Build history of the part. All positions in model axes, mm. Face numbers are marked on the shaded views. A direction names the side the tool comes from. Round coordinates to 2 decimals unless told otherwise and drop trailing zeros. Loops run counter-clockwise (first coordinate to the right, second up) from the corner with the lowest first, then second, coordinate; pieces in that order, holes last. Notation, with made-up numbers: (75, -13) - (102, -13) arc R25 cw to (102, 25) - close; hole circle Ø10 at (-7.75, -20). An arc over 180 degrees is marked (long way). Use one line per item in the form item = value. Start each with the question number.
Q1. Drill centre lines: line 1 (Y direction, x = 9, z = -1); line 2 (Z direction, x = 18, y = 40); line 3 (Y direction, x = 23, z = 0). Where is each one in solid material? Low to high.
Q2. Mould opens along X. For the marked faces 3 and 4 say: released by +X, released by -X, zero draft, split by the parting line, or undercut.
Q3. Saw through at A-A (z = 1.5). Give the cut face in (x, y).
Q4. Pin check, flat tips, straight feed: pin 1 (12 mm diameter, centred on y = 34, z = -28.5, fed in from -X); pin 2 (8 mm diameter, centred on x = -18, z = -19, fed in from +Y); pin 3 (3 mm diameter, centred on x = 15.5, y = 22.5, fed in from +Z). Stop position of each tip, or through.
Q5. Saw through at D-D (x = -40). Give the cut face in (y, z).
Q6. Saw through at C-C (y = 13). Give the cut face in (x, z).
Q7. Saw through at B-B (y = 40). Give the cut face in (x, z).
Q8. 3-axis set-ups, long thin cutter, end or side, ignore diameter. For the marked faces 1 and 2: which of +Z, -Z, +X, -X, +Y, -Y reach the whole face in a straight line?
```python
from build123d import *

# Parameters (mm, degrees)
REVOLVE1_ANGLE          = 180
SKETCH2_W               = 10
SKETCH2_H               = 40
CUT_EXTRUDE1_DEPTH      = 50
CUT_EXTRUDE2_DEPTH      = 50
CUT_EXTRUDE2_DEPTH_BACK = 50
SKETCH3_R               = 5


with BuildPart() as part:
    # Sketch1 → Revolve1 (revolve)
    with BuildSketch(Plane(origin=(0, 0, 0), x_dir=(1, 0, 0), z_dir=(0, 1, 0))):
        with BuildLine():
            Line((0, -50), (0, 50))
            ThreePointArc((0, 50), (50, 0), (0, -50))
        make_face()
    revolve(axis=Axis((0, 0, 50), (0, 0, 1)), revolution_arc=REVOLVE1_ANGLE)

    # Sketch2 → Cut-Extrude1 (cut, symmetric)
    with BuildSketch(Plane.XY):
        with Locations((5, 30)):
            Rectangle(SKETCH2_W, SKETCH2_H)
    cut_extrude1 = extrude(amount=CUT_EXTRUDE1_DEPTH, both=True, mode=Mode.SUBTRACT)

    # Mirror1: Cut-Extrude1 across plane
    add(cut_extrude1.mirror(Plane(origin=(0, 0, 0), x_dir=(0, 0, 1), z_dir=(1, 0, 0))), mode=Mode.SUBTRACT)

    # Sketch3 → Cut-Extrude2 (cut, two sides: drawn at the far end of the back side and taken through both)
    with BuildSketch(Plane(origin=(0, 0, 0), x_dir=(0, 0, -1), z_dir=(1, 0, 0)).offset(-CUT_EXTRUDE2_DEPTH_BACK)):
        with Locations(Location((0, 40, 0), (0, 0, 180))):
            Circle(SKETCH3_R)
    extrude(amount=CUT_EXTRUDE2_DEPTH + CUT_EXTRUDE2_DEPTH_BACK, mode=Mode.SUBTRACT)


solid = part.part
```
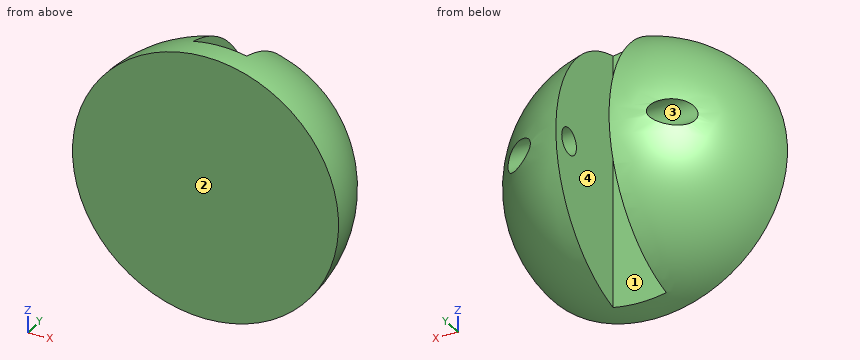
Report:
q1.line_1 = 0 to 10
q1.line_2 = -24 to -5, 5 to 24
q1.line_3 = 0 to 35
q2.face_3 = zero draft
q2.face_4 = undercut
q3.outline = (-49.98, 0) - (49.98, 0) arc R49.98 ccw to (35.45, 35.23) - (10, 35.23) - (10, 10) - (-10, 10) - (-10, 35.23) - (-35.45, 35.23) arc R49.98 ccw to start; (-22.21, 44.77) - (-10, 44.77) - (-10, 48.97) arc R49.98 ccw to start; (10, 44.77) - (22.21, 44.77) arc R49.98 ccw to (10, 48.97) - close
q4.pin_1 = -32.06
q4.pin_2 = 44.81
q4.pin_3 = 42.82
q5.outline = (0, -30) arc R30 ccw to (0, 30) - close
q6.outline = (-10, -47.23) - (-10, 47.23) arc R48.28 ccw to start; (10, -47.23) arc R48.28 ccw to (10, 47.23) - close
q7.outline = (-29.58, -5) arc R30 ccw to (-10, -28.28) - (-10, -5) - close; (-29.58, 5) - (-10, 5) - (-10, 28.28) arc R30 ccw to start; (10, -28.28) arc R30 ccw to (29.58, -5) - (10, -5) - close; (10, 5) - (29.58, 5) arc R30 ccw to (10, 28.28) - close
q8.face_1 = +Z, -Z, +Y
q8.face_2 = +Z, -Z, +X, -X, -Y
